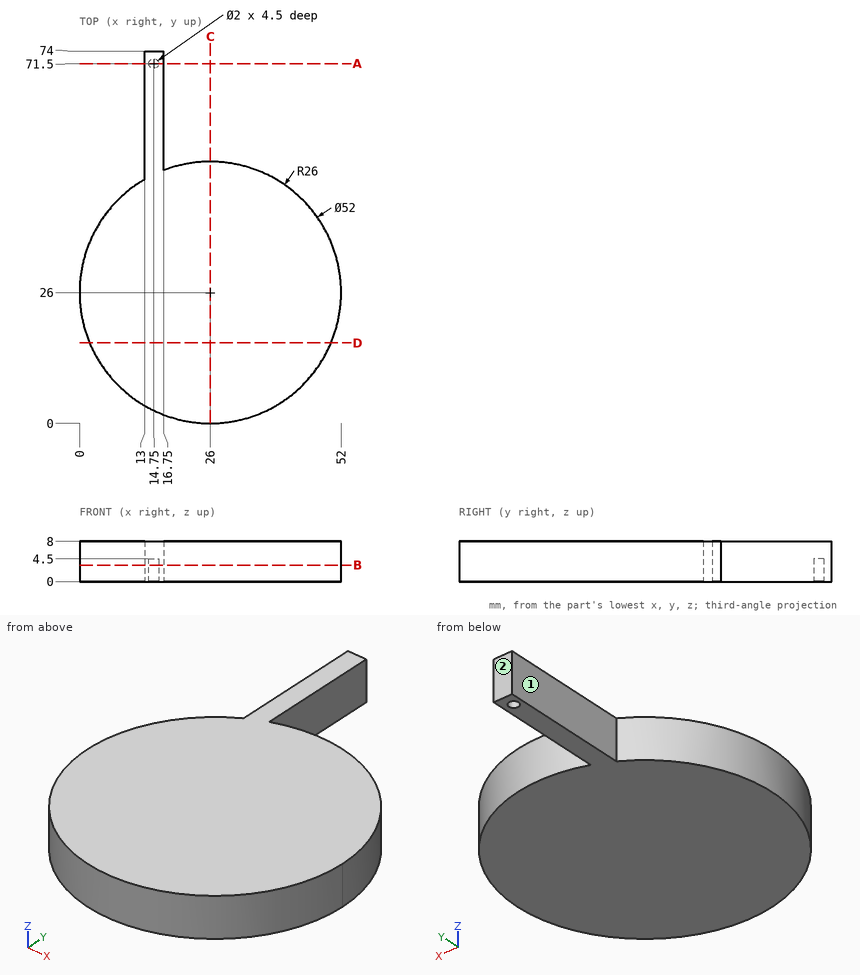
The figure shows three views and two pictorial views of one solid part (mm, origin at its lowest corner). Answer the questions. A direction names the side the tool comes from. Give positions to 0.01 mm unless a question says otherwise; leave off trailing zeros. Write each loop counter-clockwise with the first axis right and the second up, starting at its lowest first coordinate (ties: lowest second). Pieces come first, ordered by that corner, then holes.
Q1. A tool of negligible diameter and unlimited length cuts with its end or side. For the marked faces 1 and 2, from which of +Z, -Z, +X, -X, +Y, -Y can it reach the whole face along a straight path? Write none if from no direction.
Answer:
face 1: +Z, -Z, -X, +Y
face 2: +Z, -Z, +X, -X, +Y
Q2. The part is cut by section B-B on z = 3.25. Give the vertices of the cut face in (x, y).
Answer:
outline: (13, 48.52) arc R26 ccw (long way) to (16.75, 50.3) - (16.75, 74) - (13, 74) - close; hole circle Ø2 at (14.75, 71.5)
Q3. Straight lines are drawn through the part: L1, parallel to X at y = 71.5, z = 3.1; L2, parallel to Y at x = 14.75, z = 2.2; L3, parallel to Y at x = 14.5, z = 1.5. For each, find the intervals that lie inside material, in ascending order.
Answer:
L1: x = 13 to 13.75, 15.75 to 16.75
L2: y = 2.56 to 70.5, 72.5 to 74
L3: y = 2.68 to 70.53, 72.47 to 74
Q4. Given pin 1 (2.5 mm diameter, centred on y = 58.5, z = 3, fed in from -X); pin 2 (1.5 mm diameter, centred on y = 49, z = 4, fed in from +X); pin 3 (1 mm diameter, centred on x = 15, y = 71.5, fed in from -Z), each flat-ended and moving along its own axis, determine where each tip first touches the part or whether it passes through.
Answer:
pin 1: stops at x = 13
pin 2: stops at x = 39.45
pin 3: stops at z = 4.5
Q5. The part is cut by section D-D on y = 16. Give the vertices of the cut face in (x, z), and give its area (3 significant figures).
Answer:
outline: (2, 0) - (50, 0) - (50, 8) - (2, 8) - close
area: 384 mm2
Q6. The part is cut by section A-A on y = 71.5. Give the vertices of the cut face in (x, z), and give its area (3 significant figures).
Answer:
outline: (13, 0) - (13.75, 0) - (13.75, 4.5) - (15.75, 4.5) - (15.75, 0) - (16.75, 0) - (16.75, 8) - (13, 8) - close
area: 21.0 mm2
Q7. The part is cut by section C-C on x = 26. Give the vertices of the cut face in (y, z).
Answer:
outline: (0, 0) - (52, 0) - (52, 8) - (0, 8) - close
